from build123d import *

# Parameters (mm, degrees)
BOSS_EXTRUDE1_DEPTH = 2.5
SKETCH2_W           = 40
SKETCH2_H           = 55
BOSS_EXTRUDE2_DEPTH = 15
SKETCH3_W           = 32
SKETCH3_H           = 13
CUT_EXTRUDE1_DEPTH  = 146.976881731
FILLET1_R           = 5


with BuildPart() as part:
    # Sketch1 → Boss-Extrude1 (new body)
    with BuildSketch(Plane.XY):
        with BuildLine():
            ThreePointArc((88, 0), (-42.971685161, 76.794754212), (-46.032597146, -75))
            Line((-46.032597146, -75), (46.032597146, -75))
            ThreePointArc((46.032597146, -75), (76.794754212, -42.971685161), (88, 0))
        make_face()
    extrude(amount=-BOSS_EXTRUDE1_DEPTH)

    # Sketch2 → Boss-Extrude2 (add)
    with BuildSketch(Plane.XY):
        Rectangle(SKETCH2_W, SKETCH2_H)
    extrude(amount=BOSS_EXTRUDE2_DEPTH)

    # Sketch3 → Cut-Extrude1 (cut, through all)
    with BuildSketch(Plane.XZ.offset(27.5)):
        with Locations((0, 6.5)):
            Rectangle(SKETCH3_W, SKETCH3_H)
    extrude(amount=-CUT_EXTRUDE1_DEPTH, mode=Mode.SUBTRACT)

    # Fillet1
    fillet1_edges = [part.edges().sort_by_distance(p)[0] for p in [
        (-46.032597146, -75, -1.25),
        (46.032597146, -75, -1.25),
    ]]
    fillet(fillet1_edges, radius=FILLET1_R)


solid = part.part
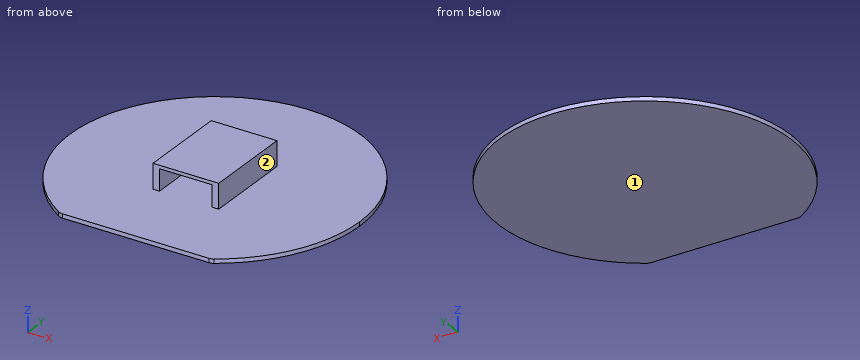
Geometry check sheet. Reference: the model listing, model coordinates, mm. Face numbers are marked on the shaded views. A direction names the side the tool comes from. Give positions to 0.01 mm unless a question says otherwise; leave off trailing zeros. Write each loop counter-clockwise with the first axis right and the second up, starting at its lowest first coordinate (ties: lowest second). Pieces come first, ordered by that corner, then holes. Notation, with made-up numbers: (2.25, -7.5) - (52.25, -7.5) arc R23 ccw to (52.25, 22.5) - close; hole circle Ø5 at (-4, -14). An arc over 180 degrees is marked (long way). Put each result on its own line as item: value.
1. Go/stop test with flat-tipped pins: pin 1 (5 mm diameter, centred on x = 43, z = 4, fed in from -Y); pin 2 (1.5 mm diameter, centred on y = -2, z = 6.5, fed in from -X); pin 3 (1 mm diameter, centred on x = -20.5, y = 58.5, fed in from +Z). Record where each tip stops, or that it passes through.
Ans:
pin 1: passes through
pin 2: stops at x = -20
pin 3: stops at z = 0
2. Sectioned sample at B-B, the plane z = 10. Enter the section's corners in (x, y), plus the area to 3 significant figures.
Ans:
outline: (-20, -27.5) - (-16, -27.5) - (-16, 27.5) - (-20, 27.5) - close; (16, -27.5) - (20, -27.5) - (20, 27.5) - (16, 27.5) - close
area: 440 mm²
3. Set-up check for the marked faces 1 and 2: record each of +Z, -Z, +X, -X, +Y, -Y from which the full face is reachable in a straight line by a thin tool's end or side.
Ans:
face 1: -Z, +X, -X, +Y, -Y
face 2: +Z, +X, +Y, -Y
4. Thickness scan on line 1 (X direction, y = 7, z = 4.5); line 2 (Z direction, x = 6.5, y = 13); line 3 (Z direction, x = -73, y = 34). Record the ranges inside material, lowest first.
Ans:
line 1: x = -20 to -16, 16 to 20
line 2: z = -2.5 to 0, 13 to 15
line 3: z = -2.5 to 0
5. Sectioned sample at D-D, the plane x = -35. Enter the section's corners in (y, z).
Ans:
outline: (-75, -2.5) - (80.74, -2.5) - (80.74, 0) - (-75, 0) - close
6. Sectioned sample at A-A, the plane x = 0. Enter the section's corners in (y, z), plus the area to 4 significant figures.
Ans:
outline: (-75, -2.5) - (88, -2.5) - (88, 0) - (-75, 0) - close; (-27.5, 13) - (27.5, 13) - (27.5, 15) - (-27.5, 15) - close
area: 517.5 mm²
7. Sectioned sample at C-C, the plane y = -21. Enter the section's corners in (x, z).
Ans:
outline: (-85.46, -2.5) - (85.46, -2.5) - (85.46, 0) - (20, 0) - (20, 15) - (-20, 15) - (-20, 0) - (-85.46, 0) - close; hole (-16, 0) - (16, 0) - (16, 13) - (-16, 13) - close
